```python
from build123d import *

# Parameters (mm, degrees)
F1_DEPTH = 25.4


with BuildPart() as f1:
    # F0 (on Front) → F1 (new body)
    with BuildSketch(Plane.XZ):
        Polygon((-101.6, -5.08), (101.6, -5.08), (101.6, 5.08), (-80.834732, 5.08), align=None)
        Polygon((101.6, 5.08), (101.6, -5.08), (215.677269, 50.735559), (194.912001, 50.735559), align=None)
        Polygon((-101.6, 5.08), (-101.6, -5.08), (-80.834732, 5.08), align=None)
        Polygon((194.912001, 50.735559), (215.677269, 50.735559), (215.677269, 60.895559), align=None)
        Polygon((12.477269, 60.895559), (-101.6, 5.08), (-80.834732, 5.08), (12.477269, 50.735559), align=None)
        Polygon((12.477269, 50.735559), (194.912001, 50.735559), (215.677269, 60.895559), (12.477269, 60.895559), align=None)
    extrude(amount=F1_DEPTH)


solid = f1.part
```
The model under review builds one solid part; all positions refer to its coordinate system, in mm. A direction names the side the tool comes from. Round coordinates to 2 decimals unless told otherwise and drop trailing zeros. Order: outer loops, then holes, each group sorted by start corner. A loop starts at its lowest first (then second) coordinate and runs counter-clockwise, first axis right, second up.
Item 1: Machinability: for faces 4 (the flat face through (148.909, -12.522, 28.227)), 5 (the flat face through (-43.76, -12.52, 33.38)), which of the approach directions +Z, -Z, +X, -X, +Y, -Y give a long, thin tool a straight path to every point of the face, cutting with its end or side? Answer none if there is none.
Working result:
face 4: +Y, -Y
face 5: +Z, -X, +Y, -Y
Item 2: Add section C-C, the plane z = 11.5. State the section outline as (x, y) points.
Working result:
outline: (-88.48, -25.4) - (-67.71, -25.4) - (-67.71, 0) - (-88.48, 0) - close; (114.72, -25.4) - (135.49, -25.4) - (135.49, 0) - (114.72, 0) - close
Item 3: Add section D-D, the plane z = 53.5. State the section outline as (x, y) points.
Working result:
outline: (-2.64, -25.4) - (215.68, -25.4) - (215.68, 0) - (-2.64, 0) - close
Item 4: For pin 1 (1.5 mm diameter, centred on x = 165, y = -19, fed in from -Z); pin 2 (8 mm diameter, centred on y = -12, z = 38.5, fed in from -X); pin 3 (3 mm diameter, centred on y = -15.5, z = 50.5, fed in from -X), all flat-tipped, find the tip position at first contact; note any pin that passes through.
Working result:
pin 1: stops at z = 25.57
pin 2: stops at x = -41.47
pin 3: stops at x = -11.84
Item 5: Add section A-A, the plane y = -20.5. State the section outline as (x, z) points, and give its area (3 significant figures).
Working result:
outline: (-101.6, -5.08) - (101.6, -5.08) - (215.68, 50.74) - (215.68, 60.9) - (12.48, 60.9) - (-101.6, 5.08) - close; hole (-80.83, 5.08) - (101.6, 5.08) - (194.91, 50.74) - (12.48, 50.74) - close
area: 6,240 mm2
Item 6: Add section B-B, the plane x = 151.5. State the section outline as (y, z) points (3 decimals).
Working result:
outline: (-25.4, 19.335) - (0, 19.335) - (0, 29.495) - (-25.4, 29.495) - close; (-25.4, 50.736) - (0, 50.736) - (0, 60.896) - (-25.4, 60.896) - close
Item 7: To check wall thickness, follow probe 1 along Z at (x, y) = (49, -13); probe 2 along Z at (x, y) = (-86.5, -4); probe 3 along X at (y, z) = (-14.75, 8.5). State the ranges of each line that lie inside material, in increasing order.
Working result:
probe 1: z = -5.08 to 5.08, 50.74 to 60.9
probe 2: z = -5.08 to 12.47
probe 3: x = -94.61 to -73.84, 108.59 to 129.36
Item 8: Draft analysis for pull direction Z (two halves, no side actions). For faces 1 (the flat face through (-34.83, -12.52, 27.59)), 2 (the flat face through (157.84, -12.522, 22.437)), 3 (the flat face through (56, 0, 55)), state which applies: released by +Z, released by -Z, zero draft, split by the parting line, or undercut.
Working result:
face 1: undercut
face 2: released by -Z
face 3: zero draft
